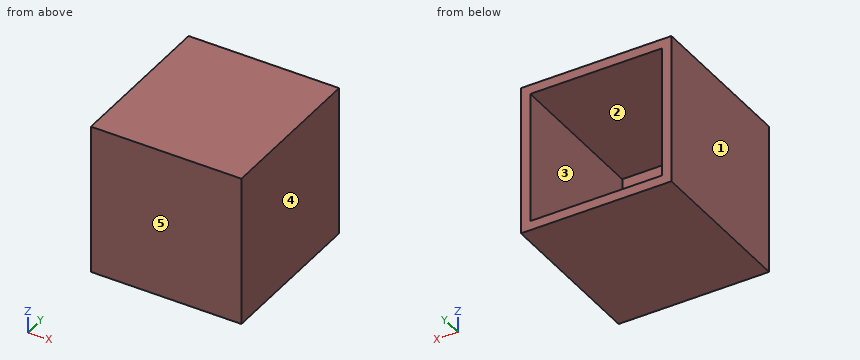
Autodesk Inventor part; units mm, degrees
ref_plane "YZ Plane" through (0, 0, 0) normal (1, 0, 0) x (0, 1, 0)
ref_plane "XZ Plane" through (0, 0, 0) normal (0, 1, 0) x (-1, 0, 0)
ref_plane "XY Plane" through (0, 0, 0) normal (0, 0, 1) x (1, 0, 0)
sketch "Sketch1" plane through (0, 0, 0) normal (0, 1, 0) x (-1, 0, 0)
  line L0 (-38.1, 38.1) -> (-38.1, -38.1)
  line L1 (-38.1, -38.1) -> (38.1, -38.1)
  line L2 (38.1, -38.1) -> (38.1, 38.1)
  line L3 (38.1, 38.1) -> (-38.1, 38.1)
  line L4 (-38.1, 38.1) -> (38.1, -38.1) construction
  line L5 (-38.1, -38.1) -> (38.1, 38.1) construction
  line L6 (-33.3375, 33.3375) -> (-33.3375, -33.3375)
  line L7 (-33.3375, -33.3375) -> (33.3375, -33.3375)
  line L8 (33.3375, -33.3375) -> (33.3375, 33.3375)
  line L9 (33.3375, 33.3375) -> (-33.3375, 33.3375)
  line L10 (-33.3375, 33.3375) -> (33.3375, -33.3375) construction
  line L11 (-33.3375, -33.3375) -> (33.3375, 33.3375) construction
  point P0 (0, 0)
  dimension "d0" = 76.2
  dimension "d1" = 4.7625
extrude "Extrusion1" add sketch "Sketch1" against normal blind 4.7625 contours L3 L2 L1 L0 | L9 L8 L7 L6
extrude "Extrusion2" add sketch "Sketch1" along normal blind 76.2
properties part number "squareMouseSupport"
Read the model definition and answer for the solid it produces. Units are mm, in the model's axes. Face numbers are marked on the shaded views. A direction names the side the tool comes from. Give positions to 0.01 mm unless a question says otherwise; leave off trailing zeros. Write each loop counter-clockwise with the first axis right and the second up, starting at its lowest first coordinate (ties: lowest second). Pieces come first, ordered by that corner, then holes. Notation, with made-up numbers: (35, 29.5) - (61, 29.5) arc R33 cw to (61, 63.5) - close; hole circle Ø3 at (22.25, 46). An arc over 180 degrees is marked (long way). Use CSV: the item, a comma, the result in double quotes. Start each with the question number.
Item 1: The part is cut by section A-A, the plane z = -5.5. Give the vertices of the cut face in (x, y).
Item 2: A flat-ended cylindrical pin translates along its axis: P1, Ø4, axis at x = -6, z = 1, coming from the +Y side. Find the tip coordinate at first contact, or state that the pin passes through.
Item 3: The mould has two halves that part along X. Classify the marked faces 3, 4 and 5: pulls with the +X half, pulls with the -X half, needs draft (parallel to the pull), parting line crosses it, or undercut.
Item 4: The part is cut by section C-C, the plane y = 6.5. Give the vertices of the cut face in (x, z), and give its area (3 significant figures).
Item 5: For the marked faces 1 and 2, determine the directions among +Z, -Z, +X, -X, +Y, -Y from which every point of the face is accessible in a straight line to the end or side of a thin tool.
Item 6: Consider line 1 (Z direction, x = 17, y = 12.5); line 2 (Y direction, x = -23, z = 33). Determine where each line is inside the solid, lowest interval first.
Item 7: The part is cut by section B-B, the plane x = -22. Give the vertices of the cut face in (y, z), and give its area (3 significant figures).
Taken from the geometry:
1,outline,"(-38.1, -4.76) - (38.1, -4.76) - (38.1, 76.2) - (33.34, 76.2) - (33.34, 0) - (-33.34, 0) - (-33.34, 76.2) - (-38.1, 76.2) - close"
2,P1,"y = 0"
3,face 3,"undercut"
3,face 4,"pulls with the +X half"
3,face 5,"needs draft"
4,outline,"(-38.1, -38.1) - (38.1, -38.1) - (38.1, 38.1) - (-38.1, 38.1) - close; hole (-33.34, -33.34) - (33.34, -33.34) - (33.34, 33.34) - (-33.34, 33.34) - close"
4,area,"1,360 mm2"
5,face 1,"+Z, -Z, -X, +Y, -Y"
5,face 2,"+Y"
6,line 1,"-38.1 to -33.34, 33.34 to 38.1"
6,line 2,"-4.76 to 0"
7,outline,"(-4.76, -38.1) - (76.2, -38.1) - (76.2, -33.34) - (0, -33.34) - (0, 33.34) - (76.2, 33.34) - (76.2, 38.1) - (-4.76, 38.1) - close"
7,area,"1,090 mm2"
